```python
from build123d import *

# Parameters (mm, degrees)
SKETCH1_R           = 60.5
SKETCH1_R_2         = 11
SKETCH1_R_3         = 1.75
SKETCH1_R_4         = 1.5
BOSS_EXTRUDE1_DEPTH = 6
SKETCH2_W           = 20
SKETCH2_H           = 15
CUT_EXTRUDE1_DEPTH  = 86.77004139
MOVE_FACE1_BY       = 0.08
MOVE_FACE1_2_BY     = 0.08
MOVE_FACE1_3_BY     = 0.08
MOVE_FACE1_4_BY     = 0.08
MOVE_FACE1_5_BY     = 0.08
MOVE_FACE1_6_BY     = 0.08
MOVE_FACE1_7_BY     = 0.08
MOVE_FACE1_8_BY     = 0.08
MOVE_FACE1_9_BY     = 0.08
MOVE_FACE1_10_BY    = 0.08
MOVE_FACE1_11_BY    = 0.08
MOVE_FACE1_12_BY    = 0.08
MOVE_FACE1_13_BY    = 0.08
MOVE_FACE1_14_BY    = 0.08
MOVE_FACE1_15_BY    = 0.08
MOVE_FACE1_16_BY    = 0.08
MOVE_FACE1_17_BY    = 0.08
MOVE_FACE1_18_BY    = 0.08
MOVE_FACE1_19_BY    = 0.08
MOVE_FACE1_20_BY    = 0.08
MOVE_FACE1_21_BY    = 0.08
MOVE_FACE1_22_BY    = 0.08
MOVE_FACE1_23_BY    = 0.08
MOVE_FACE1_24_BY    = 0.08
MOVE_FACE1_25_BY    = 0.08
MOVE_FACE1_26_BY    = 0.08


with BuildPart() as part:
    # Sketch1 → Boss-Extrude1 (new body)
    with BuildSketch(Plane.XY):
        Circle(SKETCH1_R)
        Circle(SKETCH1_R_2, mode=Mode.SUBTRACT)
        with Locations((0, -15)):
            Circle(SKETCH1_R_3, mode=Mode.SUBTRACT)
        with Locations((10.606601718, -10.606601718)):
            Circle(SKETCH1_R_4, mode=Mode.SUBTRACT)
        with Locations((0, -50)):
            Circle(SKETCH1_R_3, mode=Mode.SUBTRACT)
        with Locations((-15, 0)):
            Circle(SKETCH1_R_3, mode=Mode.SUBTRACT)
        with Locations((-10.606601718, -10.606601718)):
            Circle(SKETCH1_R_4, mode=Mode.SUBTRACT)
        with Locations((0, 15)):
            Circle(SKETCH1_R_3, mode=Mode.SUBTRACT)
        with Locations((-10.606601718, 10.606601718)):
            Circle(SKETCH1_R_4, mode=Mode.SUBTRACT)
        with Locations((10.606601718, 10.606601718)):
            Circle(SKETCH1_R_4, mode=Mode.SUBTRACT)
        with Locations((-35.355339059, -35.355339059)):
            Circle(SKETCH1_R_3, mode=Mode.SUBTRACT)
        with Locations((-50, 0)):
            Circle(SKETCH1_R_3, mode=Mode.SUBTRACT)
        with Locations((-35.355339059, 35.355339059)):
            Circle(SKETCH1_R_3, mode=Mode.SUBTRACT)
        with Locations((0, 50)):
            Circle(SKETCH1_R_3, mode=Mode.SUBTRACT)
        with Locations((50, 0)):
            Circle(SKETCH1_R_3, mode=Mode.SUBTRACT)
        with Locations((35.355339059, -35.355339059)):
            Circle(SKETCH1_R_3, mode=Mode.SUBTRACT)
    extrude(amount=BOSS_EXTRUDE1_DEPTH)

    # Sketch2 → Cut-Extrude1 (cut, through all)
    with BuildSketch(Plane.XY.offset(6)):
        Polygon((23, 14), (43, 14), (43, -26), (14.5, -26), (14.5, 9), (23, 9), align=None)
        with Locations((33, 27.5)):
            Rectangle(SKETCH2_W, SKETCH2_H)
    extrude(amount=-CUT_EXTRUDE1_DEPTH, mode=Mode.SUBTRACT)

    # Move Face1: a face moved outward by 0.08
    extrude(part.faces().sort_by_distance((23, 27.5, 3))[0], amount=MOVE_FACE1_BY, dir=(1, 0, 0))

    # Move Face1 2: a curved face moved outward by 0.08
    add(Solid.thicken(part.faces().sort_by_distance((-11, 0, 3))[0], MOVE_FACE1_2_BY))

    # Move Face1 3: a curved face moved outward by 0.08
    add(Solid.thicken(part.faces().sort_by_distance((-60.5, 0, 3))[0], MOVE_FACE1_3_BY))

    # Move Face1 4: a curved face moved outward by 0.08
    add(Solid.thicken(part.faces().sort_by_distance((-1.75, -15, 3))[0], MOVE_FACE1_4_BY))

    # Move Face1 5: a curved face moved outward by 0.08
    add(Solid.thicken(part.faces().sort_by_distance((9.106601718, -10.606601718, 3))[0], MOVE_FACE1_5_BY))

    # Move Face1 6: a curved face moved outward by 0.08
    add(Solid.thicken(part.faces().sort_by_distance((-1.75, -50, 3))[0], MOVE_FACE1_6_BY))

    # Move Face1 7: a curved face moved outward by 0.08
    add(Solid.thicken(part.faces().sort_by_distance((-16.75, 0, 3))[0], MOVE_FACE1_7_BY))

    # Move Face1 8: a curved face moved outward by 0.08
    add(Solid.thicken(part.faces().sort_by_distance((-12.106601718, -10.606601718, 3))[0], MOVE_FACE1_8_BY))

    # Move Face1 9: a curved face moved outward by 0.08
    add(Solid.thicken(part.faces().sort_by_distance((-1.75, 15, 3))[0], MOVE_FACE1_9_BY))

    # Move Face1 10: a curved face moved outward by 0.08
    add(Solid.thicken(part.faces().sort_by_distance((-12.106601718, 10.606601718, 3))[0], MOVE_FACE1_10_BY))

    # Move Face1 11: a curved face moved outward by 0.08
    add(Solid.thicken(part.faces().sort_by_distance((9.106601718, 10.606601718, 3))[0], MOVE_FACE1_11_BY))

    # Move Face1 12: a curved face moved outward by 0.08
    add(Solid.thicken(part.faces().sort_by_distance((-37.105339059, -35.355339059, 3))[0], MOVE_FACE1_12_BY))

    # Move Face1 13: a curved face moved outward by 0.08
    add(Solid.thicken(part.faces().sort_by_distance((-51.75, 0, 3))[0], MOVE_FACE1_13_BY))

    # Move Face1 14: a curved face moved outward by 0.08
    add(Solid.thicken(part.faces().sort_by_distance((-37.105339059, 35.355339059, 3))[0], MOVE_FACE1_14_BY))

    # Move Face1 15: a curved face moved outward by 0.08
    add(Solid.thicken(part.faces().sort_by_distance((-1.75, 50, 3))[0], MOVE_FACE1_15_BY))

    # Move Face1 16: a curved face moved outward by 0.08
    add(Solid.thicken(part.faces().sort_by_distance((48.25, 0, 3))[0], MOVE_FACE1_16_BY))

    # Move Face1 17: a curved face moved outward by 0.08
    add(Solid.thicken(part.faces().sort_by_distance((33.605339059, -35.355339059, 3))[0], MOVE_FACE1_17_BY))

    # Move Face1 18: a face moved outward by 0.08
    extrude(part.faces().sort_by_distance((18.75, 9, 3))[0], amount=MOVE_FACE1_18_BY, dir=(0, -1, 0))

    # Move Face1 19: a face moved outward by 0.08
    extrude(part.faces().sort_by_distance((14.5, -8.5, 3))[0], amount=MOVE_FACE1_19_BY, dir=(1, 0, 0))

    # Move Face1 20: a face moved outward by 0.08
    extrude(part.faces().sort_by_distance((28.75, -26, 3))[0], amount=MOVE_FACE1_20_BY, dir=(0, 1, 0))

    # Move Face1 21: a face moved outward by 0.08
    extrude(part.faces().sort_by_distance((43, -6, 3))[0], amount=MOVE_FACE1_21_BY, dir=(-1, 0, 0))

    # Move Face1 22: a face moved outward by 0.08
    extrude(part.faces().sort_by_distance((33, 14, 3))[0], amount=MOVE_FACE1_22_BY, dir=(0, -1, 0))

    # Move Face1 23: a face moved outward by 0.08
    extrude(part.faces().sort_by_distance((23, 11.5, 3))[0], amount=MOVE_FACE1_23_BY, dir=(1, 0, 0))

    # Move Face1 24: a face moved outward by 0.08
    extrude(part.faces().sort_by_distance((33, 20, 3))[0], amount=MOVE_FACE1_24_BY, dir=(0, 1, 0))

    # Move Face1 25: a face moved outward by 0.08
    extrude(part.faces().sort_by_distance((43, 27.5, 3))[0], amount=MOVE_FACE1_25_BY, dir=(-1, 0, 0))

    # Move Face1 26: a face moved outward by 0.08
    extrude(part.faces().sort_by_distance((33, 35, 3))[0], amount=MOVE_FACE1_26_BY, dir=(0, -1, 0))


solid = part.part
```
Input: part model. Units: mm. Frame: model coordinates. Coordinates: 2 decimals unless noted, no trailing zeros. Write each loop counter-clockwise with the first axis right and the second up, starting at its lowest first coordinate (ties: lowest second). Pieces come first, ordered by that corner, then holes. Notation, with made-up numbers: (4.5, 40.25) - (48.5, 40.25) arc R22 ccw to (48.5, 57.25) - close; hole circle Ø1 at (23.5, 38.25). An arc over 180 degrees is marked (long way). Put each result on its own line as item: value. Start each with the question number.
1) Mould query, pull axis Y, two halves, no side actions, for faces 1 (the face through (9.56, -9.647, 2.958)), 2 (the face through (-1, -13, 0)). Classes: pulls with the +Y half, pulls with the -Y half, needs draft (parallel to the pull), parting line crosses it, or undercut.
2) Cut plane D-D (z = 2.5). State how many separate pieces and enclosed holes the cut face has, plus the area to 3 significant figures.
3) Cut plane B-B (y = 0). Return the cut outline in (x, z), plus the area to 3 significant figures.
4) Cut plane A-A (x = 0). Return the cut outline in (y, z), plus the area to 3 significant figures.
5) Ray query, L1, parallel to Y at x = 0, z = 1.5; L2, parallel to Y at x = -36, z = 2.75; L3, parallel to X at y = -2.5, z = 4.65. Return the intervals inside material, ascending.
6) Cut plane C-C (x = 31). Return the cut outline in (y, z), plus the area to 3 significant figures.
7) Contact query for flat-ended pins moving along their axis: pin 1 (3 mm diameter, centred on x = 29, z = 4.5, fed in from -Y); pin 2 (1 mm diameter, centred on x = 25, z = 2, fed in from -Y); pin 3 (1.8 mm diameter, centred on x = 22.5, z = 3.5, fed in from +Y). Output: stop coordinate, or through.
Resolved:
1. face 1: undercut
1. face 2: needs draft
2. separate pieces: 1
2. enclosed holes: 17
2. area: 9,660 mm2
3. outline: (-60.58, 0) - (-51.67, 0) - (-51.67, 6) - (-60.58, 6) - close; (-48.33, 0) - (-16.67, 0) - (-16.67, 6) - (-48.33, 6) - close; (-13.33, 0) - (-10.92, 0) - (-10.92, 6) - (-13.33, 6) - close; (10.92, 0) - (14.58, 0) - (14.58, 6) - (10.92, 6) - close; (42.92, 0) - (48.33, 0) - (48.33, 6) - (42.92, 6) - close; (51.67, 0) - (60.58, 0) - (60.58, 6) - (51.67, 6) - close
3. area: 366 mm2
4. outline: (-60.58, 0) - (-51.67, 0) - (-51.67, 6) - (-60.58, 6) - close; (-48.33, 0) - (-16.67, 0) - (-16.67, 6) - (-48.33, 6) - close; (-13.33, 0) - (-10.92, 0) - (-10.92, 6) - (-13.33, 6) - close; (10.92, 0) - (13.33, 0) - (13.33, 6) - (10.92, 6) - close; (16.67, 0) - (48.33, 0) - (48.33, 6) - (16.67, 6) - close; (51.67, 0) - (60.58, 0) - (60.58, 6) - (51.67, 6) - close
4. area: 516 mm2
5. L1: y = -60.58 to -51.67, -48.33 to -16.67, -13.33 to -10.92, 10.92 to 13.33, 16.67 to 48.33, 51.67 to 60.58
5. L2: y = -48.72 to -36.9, -33.81 to 33.81, 36.9 to 48.72
5. L3: x = -60.53 to -10.63, 10.63 to 14.58, 42.92 to 60.53
6. outline: (-52.05, 0) - (-25.92, 0) - (-25.92, 6) - (-52.05, 6) - close; (13.92, 0) - (20.08, 0) - (20.08, 6) - (13.92, 6) - close; (34.92, 0) - (52.05, 0) - (52.05, 6) - (34.92, 6) - close
6. area: 296 mm2
7. pin 1: stops at y = -53.98
7. pin 2: stops at y = -55.4
7. pin 3: stops at y = 56.6
